from build123d import *

# Parameters (mm, degrees)
SKETCH1_W                      = 122
SKETCH1_H                      = 150
BOSS_EXTRUDE1_DEPTH            = 25
CBORE_FOR_M4_SHCS1_D           = 4.5
CBORE_FOR_M4_SHCS1_CBORE_D     = 8
CBORE_FOR_M4_SHCS1_CBORE_DEPTH = 4
SKETCH4_W                      = 52
SKETCH4_H                      = 13
CUT_EXTRUDE1_DEPTH             = 195.958970042
CBORE_FOR_M5_SHCS1_D           = 5.5
CBORE_FOR_M5_SHCS1_CBORE_D     = 10
CBORE_FOR_M5_SHCS1_CBORE_DEPTH = 5
CBORE_FOR_M8_SHCS1_D           = 9
CBORE_FOR_M8_SHCS1_CBORE_D     = 15
CBORE_FOR_M8_SHCS1_CBORE_DEPTH = 8


with BuildPart() as part:
    # Sketch1 → Boss-Extrude1 (new body)
    with BuildSketch(Plane.XY):
        with Locations((61, 75)):
            Rectangle(SKETCH1_W, SKETCH1_H)
    extrude(amount=BOSS_EXTRUDE1_DEPTH)

    # CBORE for M4 SHCS1 (through all)
    with Locations(Plane(origin=(4.7, 46, 25), x_dir=(1, 0, 0), z_dir=(0, 0, 1))):
        with Locations((0, 0), (26, 0), (0, -26), (26, -26), (86.6, 0), (112.6, 0), (112.6, -26), (86.6, -26)):
            CounterBoreHole(CBORE_FOR_M4_SHCS1_D / 2, CBORE_FOR_M4_SHCS1_CBORE_D / 2, CBORE_FOR_M4_SHCS1_CBORE_DEPTH)

    # Sketch4 → Cut-Extrude1 (cut, through all)
    with BuildSketch(Plane(origin=(0, 0, 0), x_dir=(1, 0, 0), z_dir=(0, 1, 0))):
        with Locations((61, -6.5)):
            Rectangle(SKETCH4_W, SKETCH4_H)
    extrude(amount=CUT_EXTRUDE1_DEPTH, mode=Mode.SUBTRACT)

    # CBORE for M5 SHCS1 (through all)
    with Locations(Plane(origin=(41, 45, 25), x_dir=(1, 0, 0), z_dir=(0, 0, 1))):
        with Locations((0, 0), (40, 0), (40, -24), (0, -24)):
            CounterBoreHole(CBORE_FOR_M5_SHCS1_D / 2, CBORE_FOR_M5_SHCS1_CBORE_D / 2, CBORE_FOR_M5_SHCS1_CBORE_DEPTH)

    # CBORE for M8 SHCS1 (through all)
    with Locations(Plane(origin=(106, 135, 0), x_dir=(-1, 0, 0), z_dir=(0, 0, -1))):
        with Locations((0, 0), (90, 0)):
            CounterBoreHole(CBORE_FOR_M8_SHCS1_D / 2, CBORE_FOR_M8_SHCS1_CBORE_D / 2, CBORE_FOR_M8_SHCS1_CBORE_DEPTH)


solid = part.part
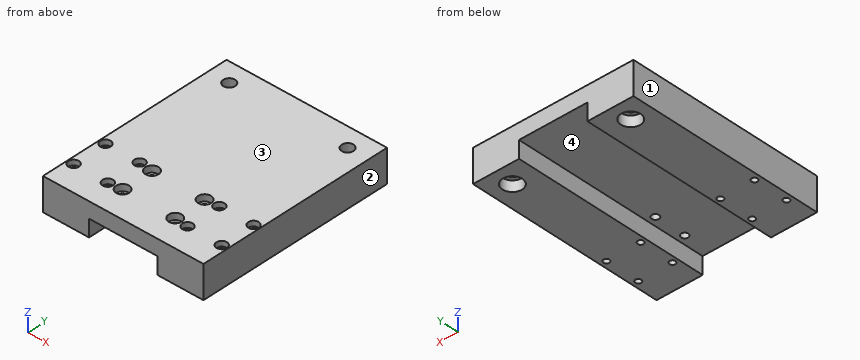
Here's how the part is built. I have some questions about the finished solid (model axes, mm). Face numbers are marked on the shaded views. Round coordinates to 2 decimals unless told otherwise and drop trailing zeros. Order: outer loops, then holes, each group sorted by start corner. A loop starts at its lowest first (then second) coordinate and runs counter-clockwise, first axis right, second up. Notation, with made-up numbers: (-26.75, 37) -> (-10.75, 37) arc R24 ccw to (-10.75, 68) -> close; hole circle Ø6 at (54, -15.5). An arc over 180 degrees is marked (long way). Return JSON: item names as keys, results as strings.
Q1. If we mould it in two halves opening along X, with no side actions, what happens to the marked faces 1, 2, 3 and 4? For each: released by +X, released by -X, zero draft, split by the parting line, or undercut.
Filled sheet:
{"face 1": "released by -X", "face 2": "released by +X", "face 3": "zero draft", "face 4": "undercut"}
Q2. If we section it at C-C on x = 91.3: List the corners of the cut face in (y, z) for me, plus the area to 3 significant figures.
Filled sheet:
{"outline": "(0, 0) -> (17.75, 0) -> (17.75, 21) -> (16, 21) -> (16, 25) -> (0, 25) -> close; (22.25, 0) -> (43.75, 0) -> (43.75, 21) -> (42, 21) -> (42, 25) -> (24, 25) -> (24, 21) -> (22.25, 21) -> close; (48.25, 0) -> (150, 0) -> (150, 25) -> (50, 25) -> (50, 21) -> (48.25, 21) -> close", "area": "3,500 mm^2"}
Q3. If we section it at B-B on x = 16: List the corners of the cut face in (y, z) for me.
Filled sheet:
{"outline": "(0, 0) -> (127.5, 0) -> (127.5, 8) -> (130.5, 8) -> (130.5, 25) -> (0, 25) -> close; (139.5, 8) -> (142.5, 8) -> (142.5, 0) -> (150, 0) -> (150, 25) -> (139.5, 25) -> close"}
Q4. For pin 1 Ø4 at (x, y) = (91.3, 46) entering from +Z; pin 2 Ø9 at (x, y) = (41, 21) entering from +Z; pin 3 Ø4 at (x, y) = (46, 106) entering from -Z, each with a flat end and sliding along its axis, tell me the tip position at first contact or that it passes through.
Filled sheet:
{"pin 1": "passes through", "pin 2": "stops at z = 20", "pin 3": "stops at z = 13"}
Q5. If we section it at D-D on y = 28.5: List the corners of the cut face in (x, z) for me, plus the area to 3 significant figures.
Filled sheet:
{"outline": "(0, 0) -> (35, 0) -> (35, 13) -> (87, 13) -> (87, 0) -> (122, 0) -> (122, 25) -> (0, 25) -> close", "area": "2,370 mm^2"}
Q6. I need wall thicknesses on line 1 along Y through (x, z) = (4.7, 22.05); line 2 along X through (y, z) = (44.5, 7); line 3 along X through (y, z) = (13.5, 7.5). Which ranges of each line are inside material? Lowest first, please. Write a range as from..to.
Filled sheet:
{"line 1": "y = 0..16, 24..42, 50..150", "line 2": "x = 0..3.02, 6.38..29.02, 32.38..35, 87..89.62, 92.98..115.62, 118.98..122", "line 3": "x = 0..35, 87..122"}
Q7. If we section it at A-A on z = 9.75: Give the number of separate pieces and of enclosed holes in the cut face, plus the area to 3 significant figures.
Filled sheet:
{"separate pieces": "2", "enclosed holes": "10", "area": "10,200 mm^2"}
